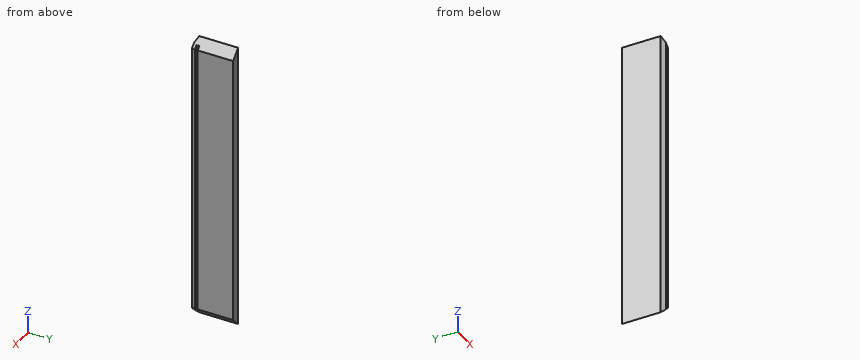
from build123d import *

# Parameters (mm, degrees)
F0_W     = 88.9
F0_H     = 609.6
F1_DEPTH = 19.05
F2_W     = 6.35
F2_H     = 609.6
F3_DEPTH = 6.35
F4_SIZE2 = 5.08
F4_SIZE  = 10.16
F6_DEPTH = 88.901


with BuildPart() as f1:
    # F0 (on Right) → F1 (new body)
    with BuildSketch(Plane.YZ):
        with Locations((44.45, 304.8)):
            Rectangle(F0_W, F0_H)
    extrude(amount=F1_DEPTH)

    # F2 (on face) → F3 (cut)
    with BuildSketch(Plane.YZ.offset(19.05)):
        with Locations((9.525, 304.8)):
            Rectangle(F2_W, F2_H)
    extrude(amount=-F3_DEPTH, mode=Mode.SUBTRACT)

    # F4
    f4_edges = [f1.edges().sort_by_distance(p)[0] for p in [
        (0, 0, 304.8),
    ]]
    chamfer(f4_edges, length=F4_SIZE, length2=F4_SIZE2)

    # F5 (on face) → F6 (cut, through all)
    with BuildSketch(Plane(origin=(0, 88.9, 0), x_dir=(-1, 0, 0), z_dir=(0, 1, 0))):
        Polygon((-19.05, 590.55), (0, 609.6), (-19.05, 609.6), align=None)
        Polygon((-19.05, 0), (0, 0), (-19.05, 19.05), align=None)
    extrude(amount=-F6_DEPTH, mode=Mode.SUBTRACT)


solid = f1.part
Geometry check sheet. Reference: the model listing, model coordinates, mm. Round coordinates to 2 decimals unless told otherwise and drop trailing zeros. Write each loop counter-clockwise with the first axis right and the second up, starting at its lowest first coordinate (ties: lowest second). Pieces come first, ordered by that corner, then holes.
Item 1: Material ranges on line 1 along Y through (x, z) = (15, 41); line 2 along X through (y, z) = (9, 360), recorded low to high.
Determined:
line 1: y = 0 to 6.35, 12.7 to 88.9
line 2: x = 0 to 12.7
Item 2: Section check A-A (z = 386). Record the boundary of the cut face in (x, y), plus the area to 3 significant figures.
Determined:
outline: (0, 5.08) - (10.16, 0) - (19.05, 0) - (19.05, 6.35) - (12.7, 6.35) - (12.7, 12.7) - (19.05, 12.7) - (19.05, 88.9) - (0, 88.9) - close
area: 1,630 mm2
Item 3: Go/stop test with a flat-tipped pin: pin 1 Ø1.9 at (y, z) = (10, 187.5) entering from +X. Record where the tip stops, or that it passes through.
Determined:
pin 1: stops at x = 12.7
Item 4: Section check B-B (y = 65). Record the boundary of the cut face in (x, z).
Determined:
outline: (0, 0) - (19.05, 19.05) - (19.05, 590.55) - (0, 609.6) - close
Item 5: Section check C-C (x = 7). Record the boundary of the cut face in (y, z), plus the area to 3 significant figures.
Determined:
outline: (1.58, 7) - (88.9, 7) - (88.9, 602.6) - (1.58, 602.6) - close
area: 52,000 mm2
